Work out the finished part from the listing and answer in its coordinate system (mm). Face numbers are marked on the shaded views. A direction names the side the tool comes from. Coordinates: 2 decimals unless noted, no trailing zeros. Write each loop counter-clockwise with the first axis right and the second up, starting at its lowest first coordinate (ties: lowest second). Pieces come first, ordered by that corner, then holes. Notation, with made-up numbers: (36.25, 4.5) - (59.25, 4.5) arc R35 cw to (59.25, 38.5) - close; hole circle Ø2 at (-27, 63.25). An arc over 180 degrees is marked (long way). One line per item, written item: value.
```python
from build123d import *

# Parameters (mm, degrees)
SKETCH1_W                    = 46
SKETCH1_H                    = 46
BOSS_EXTRUDE1_DEPTH          = 2.5
SKETCH2_W                    = 46
SKETCH2_H                    = 48.5
BOSS_EXTRUDE2_DEPTH          = 2.5
SKETCH5_W                    = 56
SKETCH5_H                    = 51
BOSS_EXTRUDE5_DEPTH          = 2.5
SKETCH6_W                    = 56
SKETCH6_H                    = 51
SKETCH6_W_2                  = 46
SKETCH6_H_2                  = 41
BOSS_EXTRUDE6_DEPTH          = 15
M2_5X0_45_TAPPED_HOLE1_D     = 2.05
M2_5X0_45_TAPPED_HOLE1_DEPTH = 4
M2_5X0_45_TAPPED_HOLE1_TIP   = 0.615882135
F_5_0MM_DOWEL_HOLE1_D        = 5
F_5_0MM_DOWEL_HOLE1_DEPTH    = 6.35
F_5_0MM_DOWEL_HOLE1_TIP      = 1.502151548
F_8_0MM_DOWEL_HOLE1_D        = 8
F_8_0MM_DOWEL_HOLE1_DEPTH    = 3
F_8_0MM_DOWEL_HOLE1_TIP      = 2.403442476
SKETCH15_W                   = 5
SKETCH15_H                   = 22.5
CUT_EXTRUDE1_DEPTH           = 15
SKETCH16_W                   = 46
SKETCH16_H                   = 2.5
CUT_EXTRUDE2_DEPTH           = 2.5
FILLET1_R                    = 3
MOVE_FACE1_BY                = 0.2
MOVE_FACE1_2_BY              = 0.2
MOVE_FACE1_3_BY              = 0.2
MOVE_FACE1_4_BY              = 0.2
MOVE_FACE1_5_BY              = 0.2
MOVE_FACE1_6_BY              = 0.2
MOVE_FACE1_7_BY              = 0.2
MOVE_FACE1_8_BY              = 0.2
MOVE_FACE2_BY                = 0.2
MOVE_FACE2_2_BY              = 0.2
M2_5X0_45_TAPPED_HOLE2_D     = 2.05
M2_5X0_45_TAPPED_HOLE2_DEPTH = 5
M2_5X0_45_TAPPED_HOLE2_TIP   = 0.615882135
SKETCH20_W                   = 9
SKETCH20_H                   = 3.5
CUT_EXTRUDE4_DEPTH           = 75.846509605
SKETCH21_W                   = 11
SKETCH21_H                   = 8
CUT_EXTRUDE5_DEPTH           = 4
MOVE_START                   = -0.1
MOVE_FACE3_OUTLINE_R         = 2.5
MOVE_FACE3_DEPTH             = 0.1
MOVE_START_2                 = 46
MOVE_FACE3_2_OUTLINE_W       = 3.5
MOVE_FACE3_2_OUTLINE_H       = 9
MOVE_FACE3_2_DEPTH           = 0.1
SKETCH17_W                   = 36
SKETCH17_H                   = 5
CUT_EXTRUDE7_DEPTH           = 12
BOSS_EXTRUDE7_START          = 5
BOSS_EXTRUDE7_DEPTH          = 36.1


# Read off the part's stored shape, not the designer's step: Move Face3
with BuildPart() as part:
    # Sketch1 → Boss-Extrude1 (new body)
    with BuildSketch(Plane(origin=(0, 0, 0), x_dir=(1, 0, 0), z_dir=(0, 1, 0))):
        with Locations((23, 23)):
            Rectangle(SKETCH1_W, SKETCH1_H)
    extrude(amount=BOSS_EXTRUDE1_DEPTH)

    # Sketch2 → Boss-Extrude2 (add)
    with BuildSketch(Plane.XZ):
        with Locations((23, -24.25)):
            Rectangle(SKETCH2_W, SKETCH2_H)
    extrude(amount=BOSS_EXTRUDE2_DEPTH)

    # Sketch5 → Boss-Extrude5 (add)
    with BuildSketch(Plane(origin=(0, 2.5, 0), x_dir=(1, 0, 0), z_dir=(0, 1, 0))):
        with Locations((23, 25.5)):
            Rectangle(SKETCH5_W, SKETCH5_H)
    extrude(amount=BOSS_EXTRUDE5_DEPTH)

    # Sketch6 → Boss-Extrude6 (add)
    with BuildSketch(Plane(origin=(0, 5, 0), x_dir=(1, 0, 0), z_dir=(0, 1, 0))):
        with Locations((23, 25.5)):
            Rectangle(SKETCH6_W, SKETCH6_H)
        with Locations((23, 25.5)):
            Rectangle(SKETCH6_W_2, SKETCH6_H_2, mode=Mode.SUBTRACT)
    extrude(amount=BOSS_EXTRUDE6_DEPTH)

    # M2.5x0.45 Tapped Hole1
    with Locations(Plane(origin=(0, 5, 0), x_dir=(1, 0, 0), z_dir=(0, 1, 0))):
        with Locations((43.4, 43.4), (28.16, 43.4), (28.16, 29.43), (43.4, 29.43)):
            Hole(M2_5X0_45_TAPPED_HOLE1_D / 2, depth=M2_5X0_45_TAPPED_HOLE1_DEPTH)
            with Locations((0, 0, -(M2_5X0_45_TAPPED_HOLE1_DEPTH + M2_5X0_45_TAPPED_HOLE1_TIP / 2))):  # 118° drill point
                Cone(0, M2_5X0_45_TAPPED_HOLE1_D / 2, M2_5X0_45_TAPPED_HOLE1_TIP, mode=Mode.SUBTRACT)

    # Ø5.0mm Dowel Hole1
    with Locations(Plane(origin=(0, 0, 0), x_dir=(0, 0, -1), z_dir=(1, 0, 0))):
        with Locations((36, 12.5)):
            Hole(F_5_0MM_DOWEL_HOLE1_D / 2, depth=F_5_0MM_DOWEL_HOLE1_DEPTH)
            with Locations((0, 0, -(F_5_0MM_DOWEL_HOLE1_DEPTH + F_5_0MM_DOWEL_HOLE1_TIP / 2))):  # 118° drill point
                Cone(0, F_5_0MM_DOWEL_HOLE1_D / 2, F_5_0MM_DOWEL_HOLE1_TIP, mode=Mode.SUBTRACT)

    # Ø8.0mm Dowel Hole1
    with Locations(Plane.ZY.offset(5)):
        with Locations((-36, 12.5)):
            Hole(F_8_0MM_DOWEL_HOLE1_D / 2, depth=F_8_0MM_DOWEL_HOLE1_DEPTH)
            with Locations((0, 0, -(F_8_0MM_DOWEL_HOLE1_DEPTH + F_8_0MM_DOWEL_HOLE1_TIP / 2))):  # 118° drill point
                Cone(0, F_8_0MM_DOWEL_HOLE1_D / 2, F_8_0MM_DOWEL_HOLE1_TIP, mode=Mode.SUBTRACT)

    # Sketch15 → Cut-Extrude1 (cut)
    with BuildSketch(Plane.XY):
        with Locations((43.5, 8.75)):
            Rectangle(SKETCH15_W, SKETCH15_H)
        with Locations((2.5, 8.75)):
            Rectangle(SKETCH15_W, SKETCH15_H)
    extrude(amount=-CUT_EXTRUDE1_DEPTH, mode=Mode.SUBTRACT)

    # Sketch16 → Cut-Extrude2 (cut)
    with BuildSketch(Plane.XY.offset(-46)):
        with Locations((23, 16.25)):
            Rectangle(SKETCH16_W, SKETCH16_H)
    extrude(amount=-CUT_EXTRUDE2_DEPTH, mode=Mode.SUBTRACT)

    # Fillet1
    fillet1_edges = [part.edges().sort_by_distance(p)[0] for p in [
        (-5, 11.25, -51),
        (51, 11.25, -51),
    ]]
    fillet(fillet1_edges, radius=FILLET1_R)

    # Move Face1: a face moved inward by 0.2
    extrude(part.faces().sort_by_distance((23, -2.5, -25.457352235))[0], amount=MOVE_FACE1_BY, dir=(0, 1, 0), mode=Mode.SUBTRACT)

    # Move Face1 2: a face moved inward by 0.2
    extrude(part.faces().sort_by_distance((23, 16.25, -48.5))[0], amount=MOVE_FACE1_2_BY, dir=(0, 0, -1), mode=Mode.SUBTRACT)

    # Move Face1 3: a face moved inward by 0.2
    extrude(part.faces().sort_by_distance((23, 17.5, -47.25))[0], amount=MOVE_FACE1_3_BY, dir=(0, 1, 0), mode=Mode.SUBTRACT)

    # Move Face1 4: a face moved inward by 0.2
    extrude(part.faces().sort_by_distance((23, 18.75, -46))[0], amount=MOVE_FACE1_4_BY, dir=(0, 0, -1), mode=Mode.SUBTRACT)

    # Move Face1 5: a face moved inward by 0.2
    extrude(part.faces().sort_by_distance((23, 0, -47.25))[0], amount=MOVE_FACE1_5_BY, dir=(0, -1, 0), mode=Mode.SUBTRACT)

    # Move Face1 6: a face moved inward by 0.2
    extrude(part.faces().sort_by_distance((23, 1.25, -46))[0], amount=MOVE_FACE1_6_BY, dir=(0, 0, 1), mode=Mode.SUBTRACT)

    # Move Face1 7: a face moved inward by 0.2
    extrude(part.faces().sort_by_distance((23, -1.25, -48.5))[0], amount=MOVE_FACE1_7_BY, dir=(0, 0, 1), mode=Mode.SUBTRACT)

    # Move Face1 8: a face moved inward by 0.2
    extrude(part.faces().sort_by_distance((23, 15, -47.25))[0], amount=MOVE_FACE1_8_BY, dir=(0, -1, 0), mode=Mode.SUBTRACT)

    # Move Face2: a face moved inward by 0.2
    extrude(part.faces().sort_by_distance((46, 0.053703704, -30.970987654))[0], amount=MOVE_FACE2_BY, dir=(-1, 0, 0), mode=Mode.SUBTRACT)

    # Move Face2 2: a face moved inward by 0.2
    extrude(part.faces().sort_by_distance((0, 0.053703704, -30.970987654))[0], amount=MOVE_FACE2_2_BY, dir=(1, 0, 0), mode=Mode.SUBTRACT)

    # M2.5x0.45 Tapped Hole2
    with Locations(Plane.XY):
        with Locations((10, 0.7), (36, 0.7)):
            Hole(M2_5X0_45_TAPPED_HOLE2_D / 2, depth=M2_5X0_45_TAPPED_HOLE2_DEPTH)
            with Locations((0, 0, -(M2_5X0_45_TAPPED_HOLE2_DEPTH + M2_5X0_45_TAPPED_HOLE2_TIP / 2))):  # 118° drill point
                Cone(0, M2_5X0_45_TAPPED_HOLE2_D / 2, M2_5X0_45_TAPPED_HOLE2_TIP, mode=Mode.SUBTRACT)

    # Sketch20 → Cut-Extrude4 (cut, through all)
    with BuildSketch(Plane.ZY.offset(-46)):
        with Locations((-36.415, 8.4)):
            Rectangle(SKETCH20_W, SKETCH20_H)
    extrude(amount=-CUT_EXTRUDE4_DEPTH, mode=Mode.SUBTRACT)

    # Sketch21 → Cut-Extrude5 (cut)
    with BuildSketch(Plane(origin=(51, 0, 0), x_dir=(0, 0, -1), z_dir=(1, 0, 0))):
        with Locations((36.415, 8.4)):
            Rectangle(SKETCH21_W, SKETCH21_H)
    extrude(amount=-CUT_EXTRUDE5_DEPTH, mode=Mode.SUBTRACT)

    # Move Face3 outline → Move Face3 (cut)
    with BuildSketch(Plane.YZ.offset(MOVE_START)):
        Polygon((5, -46), (14.8, -46), (14.8, -48.7), (17.7, -48.7), (17.7, -46.2), (20, -46.2), (20, 0), (2.5, 0), (2.5, -15), (5, -15), align=None)
        with Locations((12.5, -36)):
            Circle(MOVE_FACE3_OUTLINE_R, mode=Mode.SUBTRACT)
    extrude(amount=MOVE_FACE3_DEPTH, mode=Mode.SUBTRACT)

    # Move Face3 2 outline → Move Face3 2 (cut)
    with BuildSketch(Plane.YZ.offset(MOVE_START_2)):
        Polygon((5, -46), (14.8, -46), (14.8, -48.7), (17.7, -48.7), (17.7, -46.2), (20, -46.2), (20, 0), (2.5, 0), (2.5, -15), (5, -15), align=None)
        with Locations((8.4, -36.415)):
            Rectangle(MOVE_FACE3_2_OUTLINE_W, MOVE_FACE3_2_OUTLINE_H, mode=Mode.SUBTRACT)
    extrude(amount=MOVE_FACE3_2_DEPTH, mode=Mode.SUBTRACT)

    # Sketch17 → Cut-Extrude7 (cut)
    with BuildSketch(Plane(origin=(0, 20, 0), x_dir=(1, 0, 0), z_dir=(0, 1, 0))):
        with Locations((23, 2.5)):
            Rectangle(SKETCH17_W, SKETCH17_H)
    extrude(amount=-CUT_EXTRUDE7_DEPTH, mode=Mode.SUBTRACT)

    # Sketch8 → Boss-Extrude7 (add)
    with BuildSketch(Plane.ZY.offset(-46).offset(BOSS_EXTRUDE7_START)):
        Polygon((-22, 5), (-24.5, 5), (-22, 7), align=None)
    extrude(amount=BOSS_EXTRUDE7_DEPTH)


solid = part.part
```
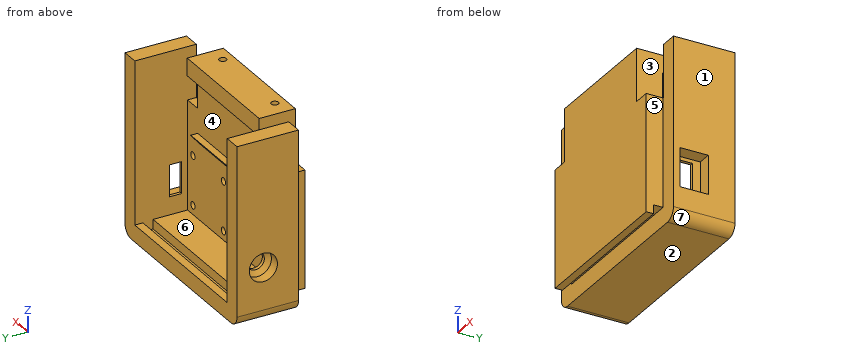
Item 1: Section A-A, the plane z = -36 is taken. Determine the outline of the cut face in (x, y).
Evaluation:
outline: (-5, 2.5) - (0.2, 2.5) - (0.2, -2.3) - (45.8, -2.3) - (45.8, 2.5) - (51, 2.5) - (51, 4.4) - (47, 4.4) - (47, 6.65) - (46.1, 6.65) - (46.1, 5) - (-0.1, 5) - (-0.1, 10) - (-1.1, 10) - (-2, 8.5) - (-5, 8.5) - close; (-5, 16.5) - (-2, 16.5) - (-1.1, 15) - (-0.1, 15) - (-0.1, 20) - (-5, 20) - close; (46.1, 10.15) - (47, 10.15) - (47, 12.4) - (51, 12.4) - (51, 20) - (46.1, 20) - close
Item 2: Determine the mould class of the marked faces 1, 2, 3 and 4 for opening direction X: +X half, -X half, draft (parallel to the pull), parting line (faces both ways), or undercut.
Evaluation:
face 1: +X half
face 2: draft
face 3: undercut
face 4: undercut
Item 3: Section B-B, the plane z = -19 is taken. Determine the outline of the cut face in (x, y).
Evaluation:
outline: (-5, 2.5) - (0.2, 2.5) - (0.2, -2.3) - (45.8, -2.3) - (45.8, 2.5) - (51, 2.5) - (51, 20) - (46.1, 20) - (46.1, 5) - (-0.1, 5) - (-0.1, 20) - (-5, 20) - close
Item 4: Consider probe 1 along X at (y, z) = (0.7, -3.35) (3 decimals); probe 2 along Y at (x, z) = (41, -48); probe 3 along Z at (x, y) = (43.4, 4.05) (3 decimals). Determine where each line is inside the solid, lowest interval first.
Evaluation:
probe 1: x = 5 to 8.975, 11.025 to 34.975, 37.025 to 41
probe 2: y = -2.3 to -0.2, 2.5 to 14.8, 17.7 to 20
probe 3: z = -51 to -44.425, -42.375 to -30.455, -28.405 to -15
Item 5: Which of the six approach directions +Z, -Z, +X, -X, +Y, -Y give full straight-line access (tool end or side, diameter ignored) to the marked faces 5, 6 and 7?
Evaluation:
face 5: +Z, -Z, +X, -Y
face 6: +Y
face 7: -Z, +X, +Y, -Y
Item 6: Section C-C, the plane x = 8 is taken. Determine the outline of the cut face in (y, z), then the cut area to 3 significant figures.
Evaluation:
outline: (-2.3, -48.3) - (-0.2, -48.3) - (-0.2, -45.8) - (2.5, -45.8) - (2.5, -51) - (20, -51) - (20, -46.2) - (17.7, -46.2) - (17.7, -48.7) - (14.8, -48.7) - (14.8, -46) - (5, -46) - (5, -24.5) - (7, -22) - (5, -22) - (5, -5) - (8, -5) - (8, 0) - (-2.3, 0) - close
area: 437 mm2
Item 7: Given pin 1 (2.5 mm diameter, centred on x = 29, y = 18.5, fed in from +Z); pin 2 (4.5 mm diameter, centred on y = 12.5, z = -36, fed in from -X); pin 3 (1.2 mm diameter, centred on x = 36, y = 0.7, fed in from +Z), each flat-ended and moving along its own axis, determine where each tip first touches the part or whether it passes through.
Evaluation:
pin 1: stops at z = -46.2
pin 2: stops at x = 46.1
pin 3: stops at z = -5.26
Item 8: Section D-D, the plane z = -9 is taken. Determine the outline of the cut face in (x, y).
Evaluation:
outline: (-5, 2.5) - (-0.1, 2.5) - (-0.1, 20) - (-5, 20) - close; (5, -2.3) - (41, -2.3) - (41, 5) - (5, 5) - close; (46.1, 2.5) - (51, 2.5) - (51, 20) - (46.1, 20) - close
